Geometry check sheet. Reference: the model listing, model coordinates, mm. A direction names the side the tool comes from. Round coordinates to 2 decimals unless told otherwise and drop trailing zeros. Write each loop counter-clockwise with the first axis right and the second up, starting at its lowest first coordinate (ties: lowest second). Pieces come first, ordered by that corner, then holes. Notation, with made-up numbers: M 81,24 L 87,24 A28 cw 87,59 Z; hole C 32,-30 d10. An arc over 180 degrees is marked long. Use a Markdown table: item, result.
```python
from build123d import *

# Parameters (mm, degrees)
SKETCH1_R           = 57.15
BOSS_EXTRUDE1_DEPTH = 12.7
CUT_EXTRUDE1_START  = -11.1125
SKETCH2_R           = 57.15
SKETCH2_R_2         = 55.5625
CUT_EXTRUDE1_DEPTH  = 11.1125
SKETCH3_R           = 50.8
CUT_EXTRUDE2_DEPTH  = 9.525
SKETCH4_R           = 12.7
BOSS_EXTRUDE2_DEPTH = 9.525
CUT_EXTRUDE4_DEPTH  = 12.7
CHAMFER1_SIZE       = 0.79375


with BuildPart() as part:
    # Sketch1 → Boss-Extrude1 (new body)
    with BuildSketch(Plane.XY):
        Circle(SKETCH1_R)
    extrude(amount=BOSS_EXTRUDE1_DEPTH)

    # Sketch2 → Cut-Extrude1 (cut)
    with BuildSketch(Plane.XY.offset(12.7).offset(CUT_EXTRUDE1_START)):
        Circle(SKETCH2_R)
        Circle(SKETCH2_R_2, mode=Mode.SUBTRACT)
    extrude(amount=CUT_EXTRUDE1_DEPTH, mode=Mode.SUBTRACT)

    # Sketch3 → Cut-Extrude2 (cut)
    with BuildSketch(Plane(origin=(0, 0, 0), x_dir=(-1, 0, 0), z_dir=(0, 0, -1))):
        Circle(SKETCH3_R)
    extrude(amount=-CUT_EXTRUDE2_DEPTH, mode=Mode.SUBTRACT)

    # Sketch4 → Boss-Extrude2 (add)
    with BuildSketch(Plane(origin=(0, 0, 9.525), x_dir=(-1, 0, 0), z_dir=(0, 0, -1))):
        with Locations(Location((0, 0, 0), (0, 0, 180))):
            Circle(SKETCH4_R)
    extrude(amount=BOSS_EXTRUDE2_DEPTH)

    # Sketch6 → Cut-Extrude4 (cut)
    with BuildSketch(Plane(origin=(0, 0, 0), x_dir=(-1, 0, 0), z_dir=(0, 0, -1))):
        Polygon((7.332348419, 0), (3.666174209, 6.35), (-3.666174209, 6.35), (-7.332348419, 0), (-3.666174209, -6.35), (3.666174209, -6.35), align=None)
    extrude(amount=-CUT_EXTRUDE4_DEPTH, mode=Mode.SUBTRACT)

    # Chamfer1
    chamfer1_edges = [part.edges().sort_by_distance(p)[0] for p in [
        (-12.7, 0, 0),
    ]]
    chamfer(chamfer1_edges, length=CHAMFER1_SIZE)


solid = part.part
```
Item 1: Mould release check, pull along X, two halves, no side actions. Record for faces 6 (the face through (5, 5, 0)), 7 (the face through (5.86, 11.267, 5.22)), 8 (the face through (-57.095, 2.513, 0.783)): +X half, -X half, draft (parallel to the pull), parting line (faces both ways), or undercut.
Outcome:
| item | result |
|---|---|
| face 6 | draft |
| face 7 | undercut |
| face 8 | parting line |
Item 2: Go/stop test with flat-tipped pins: pin 1 (3 mm diameter, centred on y = -7, z = 4, fed in from +X); pin 2 (1 mm diameter, centred on y = -19, z = 11.5, fed in from +X); pin 3 (3.5 mm diameter, centred on x = -0.5, z = 7.5, fed in from +Y); pin 4 (1.5 mm diameter, centred on x = -1, y = 11.5, fed in from -Z). Record where each tip stops, or that it passes through.
Outcome:
| item | result |
|---|---|
| pin 1 | stops at x = 55.29 |
| pin 2 | stops at x = 52.39 |
| pin 3 | stops at y = 55.56 |
| pin 4 | stops at z = 0 |
Item 3: Material ranges on line 1 along Y through (x, z) = (0, 6.75); line 2 along Y through (x, z) = (7, 6.75); line 3 along Z through (x, y) = (32, 2.5) (3 decimals), recorded low to high. Write a range as from..to.
Outcome:
| item | result |
|---|---|
| line 1 | y = -55.56..-50.8, -12.7..-6.35, 6.35..12.7, 50.8..55.56 |
| line 2 | y = -55.12..-50.32, -10.6..-0.58, 0.58..10.6, 50.32..55.12 |
| line 3 | z = 9.525..12.7 |
Item 4: Cross-section at D-D, the plane x = -18.5. Record the cut outline in (y, z) (1 decimal), and give its area (3 significant figures).
Outcome:
| item | result |
|---|---|
| outline | M -54.1,0 L -47.3,0 L -47.3,9.5 L 47.3,9.5 L 47.3,0 L 54.1,0 L 54.1,1.6 L 52.4,1.6 L 52.4,12.7 L -52.4,12.7 L -52.4,1.6 L -54.1,1.6 Z |
| area | 435 mm2 |
Item 5: Access from +Z, -Z, +X, -X, +Y, -Y to the whole of each face (thin tool, end or side, straight path). Record for faces 1 (the face through (-7.23, 55.09, 7.07)), 2 (the face through (-38, -34, 0)), 3 (the face through (5.474, 3.219, 6.261)), 4 (the face through (-1, -12, 12.7)), 5 (the face through (11.012, -49.592, 4.696)).
Outcome:
| item | result |
|---|---|
| face 1 | +Z |
| face 2 | -Z, +X, -X, +Y, -Y |
| face 3 | +Z, -Z |
| face 4 | +Z, +X, -X, +Y, -Y |
| face 5 | -Z |
Item 6: Cross-section at A-A, the plane z = 6.5. Count the separate pieces of the cut face and the enclosed holes in it, and give its area (3 significant figures).
Outcome:
| item | result |
|---|---|
| separate pieces | 2 |
| enclosed holes | 2 |
| area | 1,960 mm2 |
Item 7: Cross-section at C-C, the plane y = -36.5. Record the cut outline in (x, z) (1 decimal).
Outcome:
| item | result |
|---|---|
| outline | M -44,0 L -35.3,0 L -35.3,9.5 L 35.3,9.5 L 35.3,0 L 44,0 L 44,1.6 L 41.9,1.6 L 41.9,12.7 L -41.9,12.7 L -41.9,1.6 L -44,1.6 Z |
